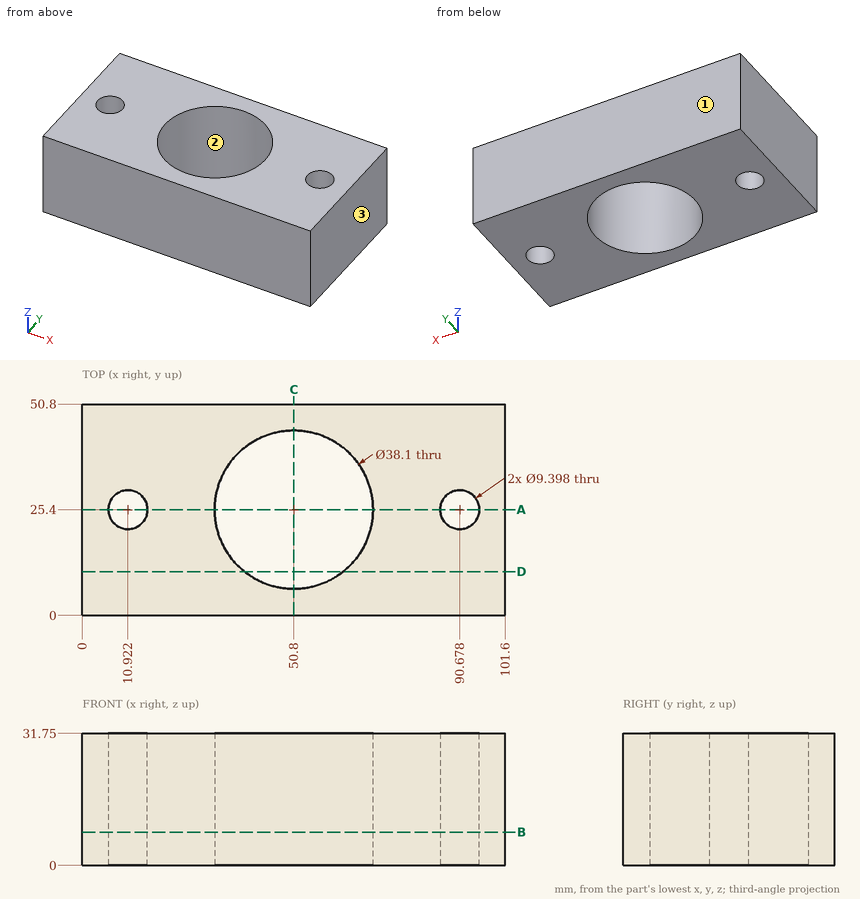
Source: three-view drawing plus pictorial views. Frame: mm from the lowest corner of the part. Give positions to 0.01 mm unless a question says otherwise; leave off trailing zeros. Loops run counter-clockwise (first coordinate to the right, second up) from the corner with the lowest first, then second, coordinate; pieces in that order, holes last. Notation, with made-up numbers: (6.5, 2.25) -> (40.5, 2.25) arc R32 ccw to (40.5, 34.25) -> close; hole circle Ø5 at (1, 18). An arc over 180 degrees is marked (long way). Put each result on its own line as item: value. Start each with the question number.
1) Cut plane B-B (z = 8). Return loops of the section in (x, y), then the cut area to 3 significant figures.
2) Contact query for a flat-ended pin moving along its axis: P1, Ø5, axis at y = 22, z = 20, coming from the -X side. Output: stop coordinate, or through.
3) Material intervals for probe 1 along X at (y, z) = (25.4, 20); probe 2 along Y at (x, z) = (50, 13); probe 3 along X at (y, z) = (23.5, 19), sorted ascending.
4) Cut plane A-A (y = 25.4). Return loops of the section in (x, z).
5) Cut plane D-D (y = 10.5). Return loops of the section in (x, z), then the cut area to 3 significant figures.
6) Cut plane C-C (x = 50.8). Return loops of the section in (y, z), then the cut area to 3 significant figures.
7) Draft query along X for the marked faces 1, 2 and 3. Return one class per face: released by +X, released by -X, zero draft, split by the parting line, or undercut.
Results are:
1. outline: (0, 0) -> (101.6, 0) -> (101.6, 50.8) -> (0, 50.8) -> close; hole circle Ø9.4 at (10.92, 25.4); hole circle Ø38.1 at (50.8, 25.4); hole circle Ø9.4 at (90.68, 25.4)
1. area: 3,880 mm2
2. P1: stops at x = 0
3. probe 1: x = 0 to 6.22, 15.62 to 31.75, 69.85 to 85.98, 95.38 to 101.6
3. probe 2: y = 0 to 6.37, 44.43 to 50.8
3. probe 3: x = 0 to 6.62, 15.22 to 31.84, 69.76 to 86.38, 94.98 to 101.6
4. outline: (0, 0) -> (6.22, 0) -> (6.22, 31.75) -> (0, 31.75) -> close; (15.62, 0) -> (31.75, 0) -> (31.75, 31.75) -> (15.62, 31.75) -> close; (69.85, 0) -> (85.98, 0) -> (85.98, 31.75) -> (69.85, 31.75) -> close; (95.38, 0) -> (101.6, 0) -> (101.6, 31.75) -> (95.38, 31.75) -> close
5. outline: (0, 0) -> (38.93, 0) -> (38.93, 31.75) -> (0, 31.75) -> close; (62.67, 0) -> (101.6, 0) -> (101.6, 31.75) -> (62.67, 31.75) -> close
5. area: 2,470 mm2
6. outline: (0, 0) -> (6.35, 0) -> (6.35, 31.75) -> (0, 31.75) -> close; (44.45, 0) -> (50.8, 0) -> (50.8, 31.75) -> (44.45, 31.75) -> close
6. area: 403 mm2
7. face 1: zero draft
7. face 2: undercut
7. face 3: released by +X
